```python
from build123d import *

# Parameters (mm, degrees)
F0_W     = 12.5
F0_H     = 14.5
F1_DEPTH = 18.2
F2_R     = 3.85
F3_DEPTH = 25
F5_DEPTH = 25


with BuildPart() as f1:
    # F0 (on Top) → F1 (new body)
    with BuildSketch(Plane.XY):
        with Locations((6.25, 7.25)):
            Rectangle(F0_W, F0_H)
    extrude(amount=F1_DEPTH)

    # F2 (on face) → F3 (cut)
    with BuildSketch(Plane.XZ):
        with Locations((6.25, 17.2)):
            Circle(F2_R)
    extrude(amount=-F3_DEPTH, mode=Mode.SUBTRACT)

    # F4 (on face) → F5 (cut)
    with BuildSketch(Plane(origin=(0, 0, 0), x_dir=(0, -1, 0), z_dir=(-1, 0, 0))):
        with BuildLine():
            Line((-11, 18.2), (-9.280318, 13.152826))
            ThreePointArc((-9.280318, 13.152826), (-7.25, 6.25), (-5.219682, 13.152826))
            Line((-5.219682, 13.152826), (-3.5, 18.2))
            Line((-3.5, 18.2), (-11, 18.2))
        make_face()
    extrude(amount=-F5_DEPTH, mode=Mode.SUBTRACT)


solid = f1.part
```
Part model, mm, in its own coordinate system. A direction names the side the tool comes from. Coordinates: 2 decimals unless noted, no trailing zeros. Order: outer loops, then holes, each group sorted by start corner. A loop starts at its lowest first (then second) coordinate and runs counter-clockwise, first axis right, second up. Notation, with made-up numbers: (16, 85.25) - (44, 85.25) arc R18 ccw to (44, 90.25) - close; hole circle Ø3 at (68.25, 74). An arc over 180 degrees is marked (long way). Return JSON: item names as keys, results as strings. Group by question number.
Item 1: Cut at A-A (z = 10). List the corners of the cut face in (x, y).
Item 2: Which spindle directions (+Z, -Z, +X, -X, +Y, -Y) get a long thin tool onto all of the face, cutting with end or side? Do faces 1 (the face through (4.77, 9.39, 13.47)), 2 (the face through (11, 13, 18.2)). Say none if no direction does.
Item 3: Cut at D-D (y = 12.75). List the corners of the cut face in (x, z), plus the area to 3 significant figures.
Item 4: Cut at C-C (z = 17.2). List the corners of the cut face in (x, y), plus the area to 3 significant figures.
Item 5: Pin check, flat tip, straight feed: pin 1 (7 mm diameter, centred on y = 7.25, z = 10, fed in from -X). Stop position of the tip, or through.
Item 6: Cut at B-B (y = 4.5). List the corners of the cut face in (x, z), plus the area to 3 significant figures.
Item 7: Drill centre lines: probe 1 along X at (y, z) = (12.1, 17.2); probe 2 along Y at (x, z) = (4, 10); probe 3 along Y at (x, z) = (1.25, 11). Where is each one in solid material? Low to high. Write a range as from..to.
Item 8: Pull direction Z, two halves, no side cores. Call faces 3 (the face through (1, 2, 18.2)), 4 (the face through (6.15, 2.54, 13.35)), 5 (the face through (6, 0, 9)): pulls with the +Z half, pulls with the -Z half, needs draft (parallel to the pull), parting line crosses it, or undercut.
Check values:
{
 "1": {"outline": "(0, 0) - (12.5, 0) - (12.5, 3.5) - (0, 3.5) - close; (0, 11) - (12.5, 11) - (12.5, 14.5) - (0, 14.5) - close"},
 "2": {"face 1": "+Z, +X, -X", "face 2": "+Z, +X, -X, +Y, -Y"},
 "3": {"outline": "(0, 0) - (12.5, 0) - (12.5, 18.2) - (9.97, 18.2) arc R3.85 cw (long way) to (2.53, 18.2) - (0, 18.2) - close", "area": "197 mm2"},
 "4": {"outline": "(0, 0) - (2.4, 0) - (2.4, 3.84) - (0, 3.84) - close; (0, 10.66) - (2.4, 10.66) - (2.4, 14.5) - (0, 14.5) - close; (10.1, 0) - (12.5, 0) - (12.5, 3.84) - (10.1, 3.84) - close; (10.1, 10.66) - (12.5, 10.66) - (12.5, 14.5) - (10.1, 14.5) - close", "area": "36.9 mm2"},
 "5": {"pin 1": "passes through"},
 "6": {"outline": "(0, 0) - (12.5, 0) - (12.5, 7.45) - (0, 7.45) - close; (0, 12.55) - (12.5, 12.55) - (12.5, 15.27) - (9.58, 15.27) arc R3.85 cw to (2.92, 15.27) - (0, 15.27) - close", "area": "118 mm2"},
 "7": {"probe 1": "x = 0..2.4, 10.1..12.5", "probe 2": "y = 0..3.5, 11..14.5", "probe 3": "y = 0..3.64, 10.86..14.5"},
 "8": {"face 3": "pulls with the +Z half", "face 4": "undercut", "face 5": "needs draft"}
}
